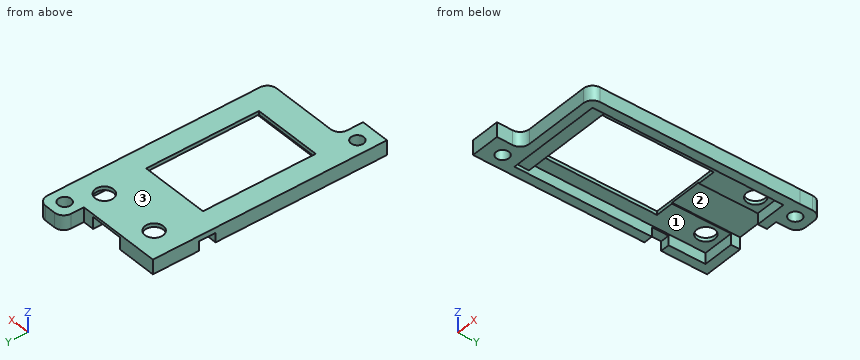
```python
from build123d import *

# Parameters (mm, degrees)
SKETCH1_R           = 1.75
BOSS_EXTRUDE1_DEPTH = 1
SKETCH2_R           = 1.75
BOSS_EXTRUDE2_DEPTH = 2
SKETCH3_R           = 2.5
SKETCH3_R_2         = 1.75
SKETCH3_W           = 19
SKETCH3_H           = 31
BOSS_EXTRUDE3_DEPTH = 1
SKETCH5_W           = 3.6
SKETCH5_H           = 4.6
CUT_EXTRUDE1_DEPTH  = 21
SKETCH6_W           = 8.995193627
SKETCH6_H           = 3.264834395
CUT_EXTRUDE2_DEPTH  = 21


with BuildPart() as part:
    # Sketch1 → Boss-Extrude1 (new body)
    with BuildSketch(Plane.XY):
        with BuildLine():
            Line((-14.676171507, 8), (-6.676171507, 8))
            Line((-6.676171507, 8), (-6.676171507, 12.347767597))
            ThreePointArc((-6.676171507, 12.347767597), (-5.943059576, 14.116412996), (-4.173686267, 14.847766361))
            Line((-4.173686267, 14.847766361), (13.97122522, 14.82972857))
            ThreePointArc((13.97122522, 14.82972857), (15.740392314, 15.560875949), (16.473710392, 17.329144394))
            Line((16.473710392, 17.329144394), (16.486530072, 72.307640303))
            Line((16.486530072, 72.307640303), (16.486530072, 75.807640303))
            ThreePointArc((16.486530072, 75.807640303), (15.754297025, 77.575407256), (13.986530072, 78.307640303))
            Line((13.986530072, 78.307640303), (10.986530072, 78.307640303))
            ThreePointArc((10.986530072, 78.307640303), (9.218763119, 77.575407256), (8.486530072, 75.807640303))
            Line((8.486530072, 75.807640303), (8.486530072, 72.327883256))
            Line((8.486530072, 72.327883256), (-14.676171507, 72.386493441))
            Line((-14.676171507, 72.386493441), (-14.676171507, 8))
        make_face()
        with Locations((12.486998677, 74.317766997)):
            Circle(SKETCH1_R, mode=Mode.SUBTRACT)
        with Locations((-10.676171507, 12.854229471)):
            Circle(SKETCH1_R, mode=Mode.SUBTRACT)
        Polygon((-12.176171507, 17.355722839), (13.97371046, 17.329727334), (13.985948537, 69.813959694), (-12.176171507, 69.880159515), align=None, mode=Mode.SUBTRACT)
    extrude(amount=BOSS_EXTRUDE1_DEPTH)

    # Sketch2 → Boss-Extrude2 (add)
    with BuildSketch(Plane.XY.offset(1)):
        with BuildLine():
            Line((-4.173686267, 14.847766361), (13.97122522, 14.82972857))
            ThreePointArc((13.97122522, 14.82972857), (15.740392314, 15.560875949), (16.473710392, 17.329144394))
            Line((16.473710392, 17.329144394), (16.486530072, 72.307640303))
            Line((16.486530072, 72.307640303), (16.486530072, 75.807640303))
            ThreePointArc((16.486530072, 75.807640303), (15.754297025, 77.575407256), (13.986530072, 78.307640303))
            Line((13.986530072, 78.307640303), (10.986530072, 78.307640303))
            ThreePointArc((10.986530072, 78.307640303), (9.218763119, 77.575407256), (8.486530072, 75.807640303))
            Line((8.486530072, 75.807640303), (8.486530072, 72.327883256))
            Line((8.486530072, 72.327883256), (-14.676171507, 72.386493441))
            Line((-14.676171507, 72.386493441), (-14.676171507, 8))
            Line((-14.676171507, 8), (-6.676171507, 8))
            Line((-6.676171507, 8), (-6.676171507, 12.347767597))
            ThreePointArc((-6.676171507, 12.347767597), (-5.943059576, 14.116412996), (-4.173686267, 14.847766361))
        make_face()
        with Locations((12.486998677, 74.317766997)):
            Circle(SKETCH2_R, mode=Mode.SUBTRACT)
        with Locations((-10.676171507, 12.854229471)):
            Circle(SKETCH2_R, mode=Mode.SUBTRACT)
        Polygon((-12.176171507, 21.330224514), (13.974643281, 21.330224514), (13.985948537, 69.813959694), (-12.176171507, 69.880159515), align=None, mode=Mode.SUBTRACT)
    extrude(amount=BOSS_EXTRUDE2_DEPTH)

    # Sketch3 → Boss-Extrude3 (add)
    with BuildSketch(Plane.XY.offset(3)):
        with BuildLine():
            Line((-4.173686267, 14.847766361), (13.97122522, 14.82972857))
            ThreePointArc((13.97122522, 14.82972857), (15.740392314, 15.560875949), (16.473710392, 17.329144394))
            Line((16.473710392, 17.329144394), (16.486530072, 72.307640303))
            Line((16.486530072, 72.307640303), (16.486530072, 75.807640303))
            ThreePointArc((16.486530072, 75.807640303), (15.754297025, 77.575407256), (13.986530072, 78.307640303))
            Line((13.986530072, 78.307640303), (10.986530072, 78.307640303))
            ThreePointArc((10.986530072, 78.307640303), (9.218763119, 77.575407256), (8.486530072, 75.807640303))
            Line((8.486530072, 75.807640303), (8.486530072, 72.327883256))
            Line((8.486530072, 72.327883256), (-14.676171507, 72.386493441))
            Line((-14.676171507, 72.386493441), (-14.676171507, 8))
            Line((-14.676171507, 8), (-6.676171507, 8))
            Line((-6.676171507, 8), (-6.676171507, 12.347767597))
            ThreePointArc((-6.676171507, 12.347767597), (-5.943059576, 14.116412996), (-4.173686267, 14.847766361))
        make_face()
        with Locations((-7.177066698, 65.873523259)):
            Circle(SKETCH3_R, mode=Mode.SUBTRACT)
        with Locations((9.307529554, 66.02592423)):
            Circle(SKETCH3_R, mode=Mode.SUBTRACT)
        with Locations((12.486998677, 74.317766997)):
            Circle(SKETCH3_R_2, mode=Mode.SUBTRACT)
        with Locations((-10.676171507, 12.854229471)):
            Circle(SKETCH3_R_2, mode=Mode.SUBTRACT)
        with Locations((0.861995575, 38.14822724)):
            Rectangle(SKETCH3_W, SKETCH3_H, mode=Mode.SUBTRACT)
    extrude(amount=BOSS_EXTRUDE3_DEPTH)

    # Sketch5 → Cut-Extrude1 (cut)
    with BuildSketch(Plane.ZY.offset(14.676171507)):
        with Locations((0.78983946, 57.439422967)):
            Rectangle(SKETCH5_W, SKETCH5_H)
    extrude(amount=-CUT_EXTRUDE1_DEPTH, mode=Mode.SUBTRACT)

    # Sketch6 → Cut-Extrude2 (cut)
    with BuildSketch(Plane(origin=(0.183069407, 72.348894077, 0), x_dir=(0.9999967986314592, -0.0025303610084290717, 0), z_dir=(0.0025303610084290713, 0.9999967986314591, 0))):
        with Locations((0.710777389, -1.632417198)):
            Rectangle(SKETCH6_W, SKETCH6_H)
    extrude(amount=-CUT_EXTRUDE2_DEPTH, mode=Mode.SUBTRACT)


solid = part.part
```
The model under review builds one solid part; all positions refer to its coordinate system, in mm. Face numbers are marked on the shaded views. Coordinates: 2 decimals unless noted, no trailing zeros. Write each loop counter-clockwise with the first axis right and the second up, starting at its lowest first coordinate (ties: lowest second). Pieces come first, ordered by that corner, then holes.
1) Clearance check with flat-ended pins moving along their axes: pin 1 Ø2 at (x, z) = (5.5, 2.5) entering from +Y; pin 2 Ø2.5 at (x, y) = (1.5, 59) entering from -Z; pin 3 Ø1.5 at (y, z) = (54, 1.5) entering from +X. State where each tip first meets the part, or that it passes through.
2) The part is to be moulded in two halves that separate along X. For the marked faces 1, 2 and 3, say which applies: pulls with the +X half, pulls with the -X half, needs draft (parallel to the pull), parting line crosses it, or undercut.
3) We need section D-D on y = 61. State the section outline as (x, z) points.
4) To check wall thickness, follow probe 1 along X at (y, z) = (74.5, 1.95); probe 2 along X at (y, z) = (67, 2); probe 3 along Y at (x, z) = (8, 2.05). State the ranges of each line that lie inside material, in increasing order.
5) We need section B-B on z = 1.8. State the section outline as (x, y) points.
6) We need section C-C on x = 3.5. State the section outline as (y, z) points.
7) We need section A-A on y = 25. State the section outline as (x, z) points.
Answer list:
1. pin 1: stops at y = 72.34
1. pin 2: stops at z = 3.26
1. pin 3: stops at x = 16.48
2. face 1: undercut
2. face 2: undercut
2. face 3: needs draft
3. outline: (-14.68, 0) - (-12.18, 0) - (-12.18, 3) - (-3.63, 3) - (-3.63, 3.26) - (5.36, 3.26) - (5.36, 3) - (13.98, 3) - (13.98, 0) - (16.48, 0) - (16.48, 4) - (-14.68, 4) - close
4. probe 1: x = 8.49 to 10.75, 14.23 to 16.49
4. probe 2: x = -14.68 to -12.18, 13.99 to 16.49
4. probe 3: y = 14.84 to 21.33, 69.83 to 72.33
5. outline: (-14.68, 8) - (-6.68, 8) - (-6.68, 12.35) arc R2.5 cw to (-4.17, 14.85) - (13.97, 14.83) arc R2.5 ccw to (16.47, 17.33) - (16.49, 72.31) - (16.49, 75.81) arc R2.5 ccw to (13.99, 78.31) - (10.99, 78.31) arc R2.5 ccw to (8.49, 75.81) - (8.49, 72.33) - (5.39, 72.34) - (5.39, 69.84) - (13.99, 69.81) - (13.97, 21.33) - (-12.18, 21.33) - (-12.18, 55.14) - (-14.68, 55.14) - close; (-14.68, 59.74) - (-12.18, 59.74) - (-12.18, 69.88) - (-3.61, 69.86) - (-3.6, 72.36) - (-14.68, 72.39) - close; hole circle Ø3.5 at (-10.68, 12.85); hole circle Ø3.5 at (12.49, 74.32)
6. outline: (14.84, 0) - (17.34, 0) - (17.34, 1) - (21.33, 1) - (21.33, 3) - (22.65, 3) - (22.65, 4) - (14.84, 4) - close; (53.65, 3.26) - (72.34, 3.26) - (72.34, 4) - (53.65, 4) - close
7. outline: (-14.68, 0) - (-12.18, 0) - (-12.18, 3) - (-8.64, 3) - (-8.64, 4) - (-14.68, 4) - close; (10.36, 3) - (13.98, 3) - (13.98, 0) - (16.48, 0) - (16.48, 4) - (10.36, 4) - close
